Autodesk Inventor part; units mm, degrees
ref_plane "center_point_XY" through (2, 0, 0) normal (1, 0, 0) x (0, 0, -1)
ref_plane "center_point_YZ" through (2, 0, 0) normal (0, 0, -1) x (0, 1, 0)
ref_plane "center_point_ZX" through (2, 0, 0) normal (0, 1, 0) x (1, 0, 0)
sketch "Sketch_1" plane through (0, 0, 0) normal (0, 0, 1) x (1, 0, 0)
  line L0 (4, 0) -> (0, 0)
  arc A0 (0, 6.2) -> (0.2, 6) centre (0.2, 6.2) ccw
  line L1 (0.2, 6) -> (3.8, 6)
  arc A1 (3.8, 6) -> (4, 6.2) centre (3.8, 6.2) ccw
  line L2 (4, 6.2) -> (4, 6.93)
  line L3 (4, 6.93) -> (3.8, 6.93)
  line L4 (3.8, 6.93) -> (3.8, 8.35)
  line L5 (3.8, 8.35) -> (4, 8.35)
  line L6 (4, 8.35) -> (4, 8.8)
  arc A2 (4, 8.8) -> (3.8, 9) centre (3.8, 8.8) ccw
  line L7 (3.8, 9) -> (0.2, 9)
  arc A3 (0.2, 9) -> (0, 8.8) centre (0.2, 8.8) ccw
  line L8 (0, 8.8) -> (0, 8.35)
  line L9 (0, 8.35) -> (0.2, 8.35)
  line L10 (0.2, 8.35) -> (0.2, 6.93)
  line L11 (0.2, 6.93) -> (0, 6.93)
  line L12 (0, 6.93) -> (0, 6.2)
revolve "Revolution1" add sketch "Sketch_1" angle 360 about axis through (4, 0, 0) along (1, 0, 0)
ref_plane "center_point_XY" through (2, 0, 0) normal (1, 0, 0) x (0, 0, -1)
ref_plane "center_point_YZ" through (2, 0, 0) normal (0, 0, -1) x (0, 1, 0)
ref_plane "center_point_ZX" through (2, 0, 0) normal (0, 1, 0) x (1, 0, 0)
ref_plane "to_housing_XY" through (0, 0, 0) normal (1, 0, 0) x (0, 0, -1)
ref_plane "to_housing_YZ" through (0, 0, 0) normal (0, 0, -1) x (0, 1, 0)
ref_plane "to_housing_ZX" through (0, 0, 0) normal (0, 1, 0) x (1, 0, 0)
ref_plane "to_ring_XY" through (3.6, 0, 0) normal (1, 0, 0) x (0, 0, -1)
ref_plane "to_ring_YZ" through (3.6, 0, 0) normal (0, 0, -1) x (0, 1, 0)
ref_plane "to_ring_ZX" through (3.6, 0, 0) normal (0, 1, 0) x (1, 0, 0)
properties part number "B6701ZZ" material "鉄、鋳鉄"
Design review of the part built by this model. Coordinates are the model's own, in mm. A direction names the side the tool comes from. Round coordinates to 2 decimals unless told otherwise and drop trailing zeros. Write each loop counter-clockwise with the first axis right and the second up, starting at its lowest first coordinate (ties: lowest second). Pieces come first, ordered by that corner, then holes. Notation, with made-up numbers: (26, 68.25) -> (48, 68.25) arc R25 cw to (48, 98.25) -> close; hole circle Ø1 at (20.25, -32.75). An arc over 180 degrees is marked (long way). Write item = value, one per line. Start each with the question number.
1) Clearance check with flat-ended pins moving along their axes: pin 1 (1 mm diameter, centred on y = 2.5, z = -5.5, fed in from +X); pin 2 (1 mm diameter, centred on x = 1, y = 6, fed in from -Z); pin 3 (7 mm diameter, centred on y = 0, z = 0, fed in from +X); pin 4 (1.5 mm diameter, centred on x = 1.5, y = 3, fed in from -Z). State where each tip first meets the part, or that it passes through.
2) Wall thickness on probe 1 along Y at (x, z) = (2.3, 0.25); probe 2 along Z at (x, y) = (2, 0); probe 3 along Z at (x, y) = (0.15, 0): over which ranges is each line inside the solid? List them lowest first. Write a range as from..to.
3) Take a section at C-C, the plane x = 2.8. State the section outline as (y, z) points.
4) Tool access review of faces 4 (the face through (0, -7, -5)), 5 (the face through (0.2, -2, 7)): name each direction out of +Z, -Z, +X, -X, +Y, -Y from which nothing blocks a thin tool from reaching the whole face with its end or side.
5) Mouldability with a two-part tool opening along Z and no side actions: class faces 1 (the face through (3.8, -2, 7)), 2 (the face through (1.975, -1.172, -8.923)), 3 (the face through (0, -5, -4)) as +Z half, -Z half, draft (parallel to the pull), parting line (faces both ways), or undercut.
Results list:
q1.pin_1 = 4
q1.pin_2 = -7.12
q1.pin_3 = through
q1.pin_4 = -8.71
q2.probe_1 = -9..-5.99, 5.99..9
q2.probe_2 = -9..-6, 6..9
q2.probe_3 = -8.99..-8.35, -6.93..-6.01, 6.01..6.93, 8.35..8.99
q3.outline = circle Ø18 at (0, 0); hole circle Ø12 at (0, 0)
q4.face_4 = +Z, -Z, -X, +Y, -Y
q4.face_5 = -X
q5.face_1 = undercut
q5.face_2 = parting line
q5.face_3 = draft
